Verification items for the finished model (mm, model axes). Face numbers are marked on the shaded views. A direction names the side the tool comes from. Give positions to 0.01 mm unless a question says otherwise; leave off trailing zeros. Loops run counter-clockwise (first coordinate to the right, second up) from the corner with the lowest first, then second, coordinate; pieces in that order, holes last. Notation, with made-up numbers: (71, -36) -> (89, -36) arc R14 ccw to (89, -12) -> close; hole circle Ø9 at (-27.5, 65.25). An arc over 180 degrees is marked (long way). Use one line per item in the form item = value. Start each with the question number.
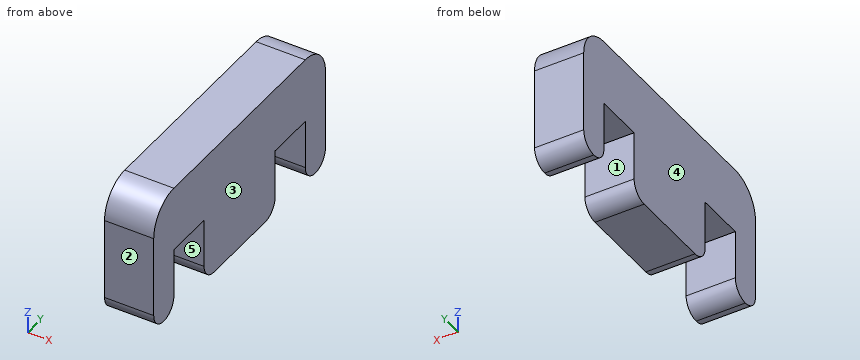
Autodesk Inventor part; units mm, degrees
ref_plane "YZ Plane" through (0, 0, 0) normal (1, 0, 0) x (0, 1, 0)
ref_plane "XZ Plane" through (0, 0, 0) normal (0, 1, 0) x (-1, 0, 0)
ref_plane "XY Plane" through (0, 0, 0) normal (0, 0, 1) x (1, 0, 0)
sketch "草圖1" plane through (0, 0, 0) normal (1, 0, 0) x (0, 1, 0)
  line L0 (-8.5245, 0) -> (-8.5245, -8)
  line L1 (-8.5245, -8) -> (-6.5245, -8)
  line L2 (-6.5245, -8) -> (-6.5245, -4)
  line L3 (-6.5245, -4) -> (-3.5245, -4)
  line L4 (3.5245, -4) -> (3.5245, -8)
  line L5 (3.5245, -8) -> (-3.5245, -8)
  line L6 (8.5245, 0) -> (8.5245, -8)
  line L7 (8.5245, -8) -> (6.5245, -8)
  line L8 (6.5245, -8) -> (6.5245, -4)
  line L9 (6.5245, -4) -> (3.5245, -4)
  line L10 (8.5245, 0) -> (-8.5245, 0)
  line L11 (-3.5245, -8) -> (-3.5245, -4)
  point P0 (0, 0)
  point P1 (0, 0)
  point P2 (0, 0)
  dimension "d2" = 3
  dimension "d3" = 7.049
  dimension "d4" = 8
  dimension "d5" = 4
  dimension "d6" = 2
  dimension "d12" = 17.049
extrude "擠出1" add sketch "草圖1" along normal blind 3
fillet "圓角1" radius 2 2 edges at (1.5, 8.5245, 0) (1.5, -8.5245, 0)
fillet "圓角2" radius 1 4 edges at (1.5, 6.5245, -8) (1.5, 3.5245, -8) (1.5, -3.5245, -8) (1.5, -6.5245, -8)
fillet "圓角3" radius 1 2 edges at (1.5, 8.5245, -8) (1.5, -8.5245, -8)
properties part number "flange support" material "木材 (楓木)"
Item 1: Sectioned sample at C-C, the plane y = 5. Enter the section's corners in (x, z), and give its area (3 significant figures).
Item 2: Draft check along Y on the marked faces 1, 2 and 3. Enter one of: +Y half, -Y half, draft (parallel to the pull), parting line (faces both ways), or undercut.
Item 3: Sectioned sample at A-A, the plane z = -6. Enter the section's corners in (x, y), and give its area (3 significant figures).
Item 4: Tool access check on the marked faces 4 and 5. Record the directions out of +Z, -Z, +X, -X, +Y, -Y that give a thin tool (end or side, any length) a straight path to the whole face; none if there is none.
Item 5: Material ranges on line 1 (Y direction, x = 1.7, z = -5.5); line 2 (Y direction, x = 1.85, z = -7.25); line 3 (Z direction, x = 1.85, y = -4.5), recorded low to high.
Item 6: Gauge pin test, flat end, axial feed: pin 1 Ø1.5 at (x, y) = (1, -5.5) entering from -Z. Record the tip position at first contact, or that the pin passes through.
Item 7: Sectioned sample at D-D, the plane z = -0.5. Enter the section's corners in (x, y).
Outcome:
q1.outline = (0, -4) -> (3, -4) -> (3, 0) -> (0, 0) -> close
q1.area = 12.0 mm^2
q2.face_1 = undercut
q2.face_2 = -Y half
q2.face_3 = draft
q3.outline = (0, -8.52) -> (3, -8.52) -> (3, -6.52) -> (0, -6.52) -> close; (0, -3.52) -> (3, -3.52) -> (3, 3.52) -> (0, 3.52) -> close; (0, 6.52) -> (3, 6.52) -> (3, 8.52) -> (0, 8.52) -> close
q3.area = 33.1 mm^2
q4.face_4 = +Z, -Z, -X, +Y, -Y
q4.face_5 = -Z, +X, -X
q5.line_1 = -8.52 to -6.52, -3.52 to 3.52, 6.52 to 8.52
q5.line_2 = -8.49 to -6.56, -3.49 to 3.49, 6.56 to 8.49
q5.line_3 = -4 to 0
q6.pin_1 = -4
q7.outline = (0, -7.85) -> (3, -7.85) -> (3, 7.85) -> (0, 7.85) -> close
